Autodesk Inventor part; units mm, degrees
ref_plane "YZ Plane" through (0, 0, 0) normal (1, 0, 0) x (0, 1, 0)
ref_plane "XZ Plane" through (0, 0, 0) normal (0, 1, 0) x (-1, 0, 0)
ref_plane "XY Plane" through (0, 0, 0) normal (0, 0, 1) x (1, 0, 0)
sketch "草圖1" plane through (0, 0, 0) normal (0, 1, 0) x (-1, 0, 0)
  line L0 (70, -124.9774) -> (-70, -124.9774)
  line L1 (-70, -124.9774) -> (-70, 55.0226)
  line L2 (-70, 55.0226) -> (70, 55.0226)
  line L3 (70, 55.0226) -> (70, -124.9774)
  point P0 (0, 0)
  point P1 (0, 55.0226)
  dimension "d0" = 140
  dimension "d1" = 180
extrude "擠出1" add sketch "草圖1" along normal blind 6
sketch "草圖2" plane through (0, 0, 0) normal (0, -1, 0) x (1, 0, 0)
  line L0 (-65, 50.0226) -> (65, 50.0226)
  line L1 (65, 50.0226) -> (65, -49.9774)
  line L2 (65, -49.9774) -> (-65, -49.9774)
  line L3 (-65, -49.9774) -> (-65, 50.0226)
  line L4 (70, 55.0226) -> (-70, 55.0226)
  line L5 (15, -54.9774) -> (-15, -54.9774)
  point P0 (0, 0)
  point P1 (0, 50.0226)
  point P2 (0, -54.9774)
  dimension "d18" = 130
  dimension "d19" = 100
  dimension "d20" = 5
  dimension "d21" = 30
  dimension "d22" = 110
hole "孔1" at (65, 0, 50.0226) at (65, 0, -49.9774) at (-65, 0, -49.9774) at (-65, 0, 50.0226) at (15, 0, -54.9774) at (-15, 0, -54.9774) direction (0, 1, 0) diameter 3.3 end through all counterbore diameter 6.5 counterbore depth 3.3
sketch "草圖3" plane through (0, 6, 0) normal (0, 1, 0) x (1, 0, 0)
  circle A0 centre (0, 94.9774) radius 22.5
  line L0 (-70, -55.0226) -> (70, -55.0226)
  point P0 (0, 0)
  dimension "d15" = 45
  dimension "d23" = 150
extrude "擠出2" cut sketch "草圖3" against normal blind 0.1
properties part number "A0005"
The model under review builds one solid part; all positions refer to its coordinate system, in mm. A direction names the side the tool comes from. Round coordinates to 2 decimals unless told otherwise and drop trailing zeros. Use CSV: the item, a comma, the result in double quotes. Start each with the question number.
(1) Tool access review of faces 1 (the face through (1, 0, -34)), 2 (the face through (-66, 3.3, 52)): name each direction out of +Z, -Z, +X, -X, +Y, -Y from which nothing blocks a thin tool from reaching the whole face with its end or side.
(2) Mouldability with a two-part tool opening along Z and no side actions: class faces 3 (the face through (-1, 3, -124.977)), 4 (the face through (1, 3, 55.023)), 5 (the face through (-70, 3, -34)), 6 (the face through (-63.76, 1.67, 47.02)) as pulls with the +Z half, pulls with the -Z half, needs draft (parallel to the pull), parting line crosses it, or undercut.
(3) Wall thickness on probe 1 along Z at (x, y) = (-65, 5.05); probe 2 along Z at (x, y) = (-15, 4.8); probe 3 along Y at (x, z) = (-12, -101.5): over which ranges is each line inside the solid? List them lowest first. Write a range as from..to.
(4) Insertion check: pin 1 (2 mm diameter, centred on x = -16.5, z = -55, fed in from -Y); pin 2 (22.5 mm diameter, centred on x = -3.5, z = -93, fed in from +Y). Each pin has a flat end and moves straight along its axis. Give the tip position at first contact, or say it passes through.
Responses:
1,face 1,"+Z, -Z, +X, -X, -Y"
1,face 2,"-Y"
2,face 3,"pulls with the -Z half"
2,face 4,"pulls with the +Z half"
2,face 5,"needs draft"
2,face 6,"undercut"
3,probe 1,"-124.98..-51.63, -48.33..48.37, 51.67..55.02"
3,probe 2,"-124.98..-56.63, -53.33..55.02"
3,probe 3,"0..5.9"
4,pin 1,"y = 3.3"
4,pin 2,"y = 5.9"
